The figure shows three views and two pictorial views of one solid part (mm, origin at its lowest corner). Answer the questions. A direction names the side the tool comes from. Coordinates: 2 decimals unless noted, no trailing zeros. Order: outer loops, then holes, each group sorted by start corner. A loop starts at its lowest first (then second) coordinate and runs counter-clockwise, first axis right, second up. Notation, with made-up numbers: (7, 65.25) -> (11, 65.25) arc R35 ccw to (11, 97.25) -> close; hole circle Ø6 at (2, 24). An arc over 180 degrees is marked (long way). Return JSON: item names as keys, results as strings. Group by question number.
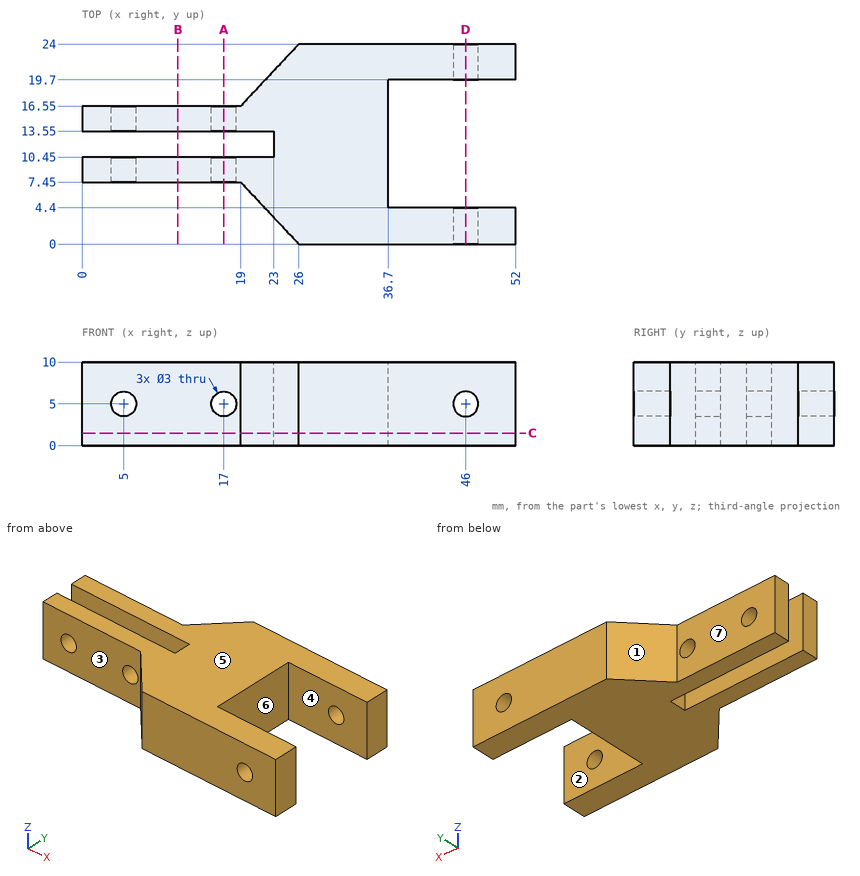
1. Find section A-A on x = 17. Determine the outline of the cut face in (y, z).
2. Find section C-C on z = 1.5. Determine the outline of the cut face in (x, y), and give its area (3 significant figures).
3. Which of the six approach directions +Z, -Z, +X, -X, +Y, -Y give full straight-line access (tool end or side, diameter ignored) to the marked faces 5, 6 and 7?
4. Find section D-D on x = 46. Determine the outline of the cut face in (y, z).
5. Find section B-B on x = 11.5. Determine the outline of the cut face in (y, z).
6. Straight lines are drawn through the part: L1, parallel to X at y = 15.3, z = 5; L2, parallel to Z at x = 46, y = 2.8; L3, parallel to Y at x = 13, z = 3.75. For each, find the intervals that lie inside material, in ascending order.
7. For a pull along Y with two mould halves and no side action, classify the marked faces 1, 2, 3 and 4 as released by +Y, released by -Y, zero draft, split by the parting line, or undercut.
8. Given pin 1 (3 mm diameter, centred on x = 6, z = 7.5, fed in from +Y); pin 2 (0.9 mm diameter, centred on y = 12, z = 3, fed in from -X); pin 3 (1 mm diameter, centred on y = 21, z = 1, fed in from -X), each flat-ended and moving along its own axis, determine where each tip first touches the part or whether it passes through.
Result:
{
 "1": {"outline": "(7.45, 0) -> (10.45, 0) -> (10.45, 3.5) -> (7.45, 3.5) -> close; (7.45, 6.5) -> (10.45, 6.5) -> (10.45, 10) -> (7.45, 10) -> close; (13.55, 0) -> (16.55, 0) -> (16.55, 3.5) -> (13.55, 3.5) -> close; (13.55, 6.5) -> (16.55, 6.5) -> (16.55, 10) -> (13.55, 10) -> close"},
 "2": {"outline": "(0, 7.45) -> (19, 7.45) -> (26, 0) -> (52, 0) -> (52, 4.4) -> (36.7, 4.4) -> (36.7, 19.7) -> (52, 19.7) -> (52, 24) -> (26, 24) -> (19, 16.55) -> (0, 16.55) -> (0, 13.55) -> (23, 13.55) -> (23, 10.45) -> (0, 10.45) -> close", "area": "607 mm^2"},
 "3": {"face 5": "+Z, +X, -X, +Y, -Y", "face 6": "+Z, -Z, +X", "face 7": "+Z, -Z, -X, +Y"},
 "4": {"outline": "(0, 0) -> (4.4, 0) -> (4.4, 3.5) -> (0, 3.5) -> close; (0, 6.5) -> (4.4, 6.5) -> (4.4, 10) -> (0, 10) -> close; (19.7, 0) -> (24, 0) -> (24, 3.5) -> (19.7, 3.5) -> close; (19.7, 6.5) -> (24, 6.5) -> (24, 10) -> (19.7, 10) -> close"},
 "5": {"outline": "(7.45, 0) -> (10.45, 0) -> (10.45, 10) -> (7.45, 10) -> close; (13.55, 0) -> (16.55, 0) -> (16.55, 10) -> (13.55, 10) -> close"},
 "6": {"L1": "0 to 3.5, 6.5 to 15.5, 18.5 to 36.7", "L2": "0 to 3.5, 6.5 to 10", "L3": "7.45 to 10.45, 13.55 to 16.55"},
 "7": {"face 1": "released by +Y", "face 2": "undercut", "face 3": "released by -Y", "face 4": "undercut"},
 "8": {"pin 1": "y = 16.55", "pin 2": "x = 23", "pin 3": "x = 22.71"}
}
